```python
from build123d import *

# Parameters (mm, degrees)
SKETCH1_W            = 23
SKETCH1_H            = 12.6
BOSS_EXTRUDE1_DEPTH  = 22.8
BOSS_EXTRUDE2_DEPTH  = 4.2
SKETCH3_R            = 2.5
SKETCH3_R_2          = 1
EXTRUDE_THIN1_DEPTH  = 4
FILLET1_R            = 1
BOSS_EXTRUDE4_START  = -4.2
BOSS_EXTRUDE4_DEPTH  = 2.5
FILLET2_R            = 1
FILLET2_OF_MIRROR1_R = 1


with BuildPart() as part:
    # Sketch1 → Boss-Extrude1 (new body)
    with BuildSketch(Plane(origin=(0, 0, 0), x_dir=(1, 0, 0), z_dir=(0, 1, 0))):
        Rectangle(SKETCH1_W, SKETCH1_H)
    extrude(amount=BOSS_EXTRUDE1_DEPTH)

    # Sketch2 → Boss-Extrude2 (add)
    with BuildSketch(Plane(origin=(0, 22.8, 0), x_dir=(1, 0, 0), z_dir=(0, 1, 0))):
        with BuildLine():
            ThreePointArc((0.172413793, -2.759859636), (11.5, 0), (0.172413793, 2.759859636))
            ThreePointArc((0.172413793, 2.759859636), (-3.1, 0), (0.172413793, -2.759859636))
        make_face()
    extrude(amount=BOSS_EXTRUDE2_DEPTH)

    # Sketch3 → Extrude-Thin1 (add)
    with BuildSketch(Plane(origin=(0, 27, 0), x_dir=(1, 0, 0), z_dir=(0, 1, 0))):
        with Locations((5.5, 0)):
            Circle(SKETCH3_R)
        with Locations((5.5, 0)):
            Circle(SKETCH3_R_2, mode=Mode.SUBTRACT)
    extrude(amount=EXTRUDE_THIN1_DEPTH)

    # Fillet1
    fillet1_edges = [part.edges().sort_by_distance(p)[0] for p in [
        (0, 0, 6.3),
        (-11.5, 0, 0),
        (0, 0, -6.3),
        (11.5, 0, 0),
        (11.5, 11.4, 6.3),
        (-11.5, 11.4, 6.3),
        (-11.5, 11.4, -6.3),
        (11.5, 11.4, -6.3),
    ]]
    fillet(fillet1_edges, radius=FILLET1_R)

    # Sketch4 → Boss-Extrude4 (add)
    with BuildSketch(Plane(origin=(0, 22.8, 0), x_dir=(1, 0, 0), z_dir=(0, 1, 0)).offset(BOSS_EXTRUDE4_START)):
        with BuildLine():
            Line((-9.107735151, 6.3), (-16, 6.3))
            Line((-16, 6.3), (-16, 0.5))
            Line((-16, 0.5), (-15.25399362, 0.5))
            ThreePointArc((-15.25399362, 0.5), (-12.65, 0), (-15.25399362, -0.5))
            Line((-15.25399362, -0.5), (-16, -0.5))
            Line((-16, -0.5), (-16, -6.3))
            Line((-16, -6.3), (-9.107735151, -6.3))
            Line((-9.107735151, -6.3), (-9.107735151, 6.3))
        make_face()
    boss_extrude4 = extrude(amount=-BOSS_EXTRUDE4_DEPTH)

    # Fillet2
    fillet2_edges = [part.edges().sort_by_distance(p)[0] for p in [
        (-16, 17.35, -6.3),
        (-16, 17.35, 6.3),
    ]]
    fillet(fillet2_edges, radius=FILLET2_R)

    # Mirror1: Boss-Extrude4 across plane
    add(boss_extrude4.mirror(Plane(origin=(0, 0, 0), x_dir=(0, 0, 1), z_dir=(1, 0, 0))))

    # Fillet2 of Mirror1
    fillet2_of_mirror1_edges = [part.edges().sort_by_distance(p)[0] for p in [
        (16, 17.35, -6.3),
        (16, 17.35, 6.3),
    ]]
    fillet(fillet2_of_mirror1_edges, radius=FILLET2_OF_MIRROR1_R)


solid = part.part
```
For this review, take the finished solid that the model builds, in its own axes (mm). A direction names the side the tool comes from. Give positions to 0.01 mm unless a question says otherwise; leave off trailing zeros. Loops run counter-clockwise (first coordinate to the right, second up) from the corner with the lowest first, then second, coordinate; pieces in that order, holes last. Notation, with made-up numbers: M -27.75,-27.5 L 8.25,-27.5 A28 cw 8.25,2.5 Z; hole C 40,-3.5 d8. An arc over 180 degrees is marked long. One line per item, written item: value. Start each with the question number.
Q1. Draft analysis for pull direction Z (two halves, no side actions). For faces 4 (the face through (0, 12, 6.3)), 5 (the face through (7.885, 28.972, -0.751)), 6 (the face through (12.65, 17.37, -0.05)), 7 (the face through (-13.9, 16.1, -1.5)), state which applies: released by +Z, released by -Z, zero draft, split by the parting line, or undercut.
Q2. For L1, parallel to X at y = 28.8, z = 0; L2, parallel to Y at x = -4.5, z = -0.25; L3, parallel to Y at x = 14, z = 3.25, list the stretches that pass through material, from the lowest coordinate up.
Q3. Machinability: for faces 1 (the face through (11.199, 20.729, -6.015)), 2 (the face through (11.5, 8, 0)), 3 (the face through (4.7, 29, 0.6)), which of the approach directions +Z, -Z, +X, -X, +Y, -Y give a long, thin tool a straight path to every point of the face, cutting with its end or side? Answer none if there is none.
Q4. Add section D-D (z = 4.5). Give the boundary of the cut face in (x, y).
Q5. Add section A-A (x = -14). Give the boundary of the cut face in (y, z), and give its area (4 significant figures).
Q6. Add section B-B (y = 8.5). Give the boundary of the cut face in (x, z), and give its area (3 significant figures).
Q7. Clearance check with flat-ended pins moving along their axes: pin 1 Ø1 at (x, z) = (6, -0.5) entering from +Y; pin 2 Ø1.5 at (y, z) = (27, -0.5) entering from +X; pin 3 Ø3.5 at (x, z) = (-14, 0) entering from -Y; pin 4 Ø0.8 at (x, y) = (15.5, 17.5) entering from -Z (3 decimals). State where each tip first meets the part, or that it passes through.
Q8. Add section C-C (x = -0.3). Give the boundary of the cut face in (y, z).
Reply:
1. face 4: released by +Z
1. face 5: split by the parting line
1. face 6: undercut
1. face 7: zero draft
2. L1: 3 to 4.5, 6.5 to 8
2. L2: 0 to 22.8
2. L3: 16.1 to 18.6
3. face 1: -Z, +X, +Y
3. face 2: +Z, -Z, +X, -Y
3. face 3: +Y
4. outline: M -16,16.1 L -11.5,16.1 L -11.5,1 A1 ccw -10.5,0 L 10.5,0 A1 ccw 11.5,1 L 11.5,16.1 L 16,16.1 L 16,18.6 L 11.5,18.6 L 11.5,22.8 L 9.47,22.8 L 9.47,27 L 1.53,27 L 1.53,22.8 L -11.5,22.8 L -11.5,18.6 L -16,18.6 Z
5. outline: M 16.1,-6.3 L 18.6,-6.3 L 18.6,-1.35 L 16.1,-1.35 Z; M 16.1,1.35 L 18.6,1.35 L 18.6,6.3 L 16.1,6.3 Z
5. area: 24.75 mm²
6. outline: M -11.5,-5.3 A1 ccw -10.5,-6.3 L 10.5,-6.3 A1 ccw 11.5,-5.3 L 11.5,5.3 A1 ccw 10.5,6.3 L -10.5,6.3 A1 ccw -11.5,5.3 Z
6. area: 289 mm²
7. pin 1: y = 31
7. pin 2: x = 11.5
7. pin 3: y = 16.1
7. pin 4: z = -6.295
8. outline: M 0,-5.3 A1 ccw 1,-6.3 L 22.8,-6.3 L 22.8,-2.8 L 27,-2.8 L 27,2.8 L 22.8,2.8 L 22.8,6.3 L 1,6.3 A1 ccw 0,5.3 Z
